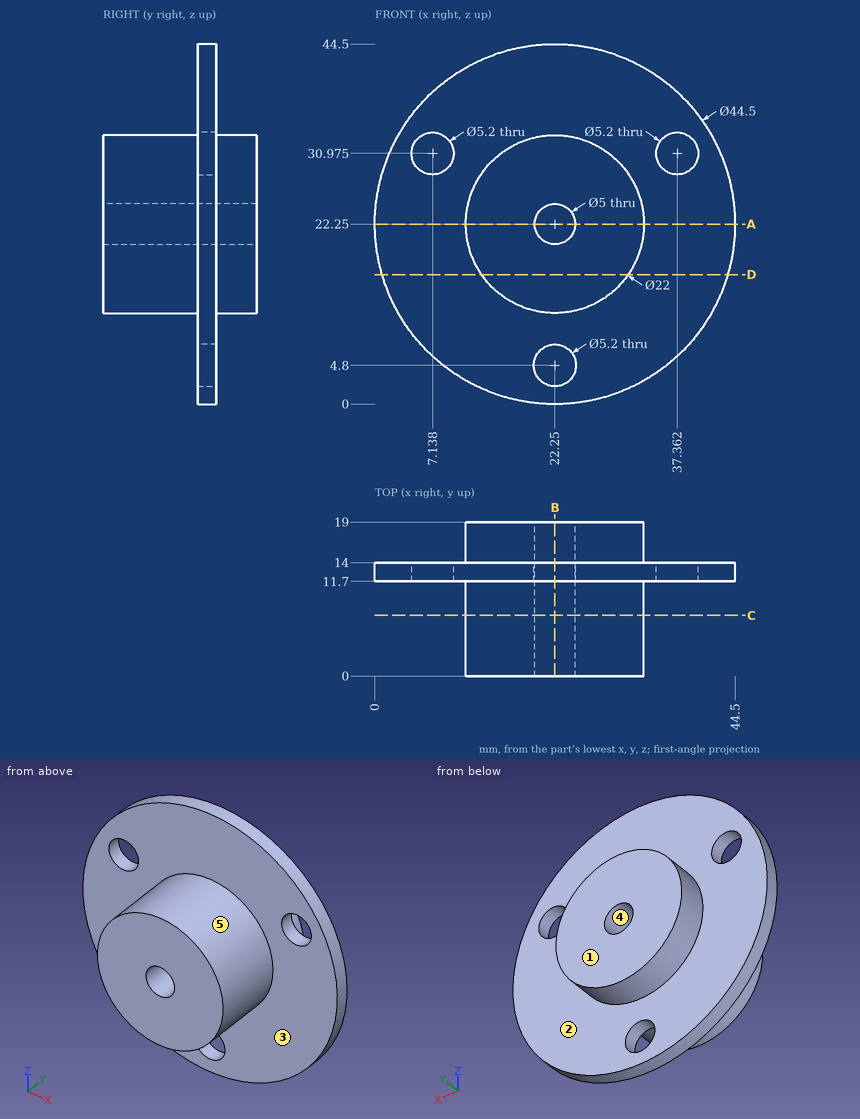
Job drawing, mm, ordinate dimensions from the low corner. One solid piece. A direction names the side the tool comes from. Give positions to 0.01 mm unless a question says otherwise; leave off trailing zeros. Order: outer loops, then holes, each group sorted by start corner. A loop starts at its lowest first (then second) coordinate and runs counter-clockwise, first axis right, second up. Notation, with made-up numbers: (52, 2) - (94, 2) arc R26 ccw to (94, 32) - close; hole circle Ø5 at (26.25, -40). An arc over 180 degrees is marked (long way). Return JSON: item names as keys, results as strings.
1) Flat gauge pins, fed straight in: P1, Ø6, axis at y = 6, z = 22, coming from the +X side; P2, Ø2, axis at y = 15.5, z = 31.5, coming from the -X side; P3, Ø10, axis at x = 10.5, y = 12.5, coming from the +Z side; P4, Ø8, axis at x = 22.25, z = 22.25, coming from the -Y side. Where does each tip first touch, or does it go through?
Geometry says:
{"P1": "x = 33.25", "P2": "x = 14.97", "P3": "z = 43.45", "P4": "y = 0"}
2) Cut at A-A, the plane z = 22.25. Give the cut face in (x, y).
Geometry says:
{"outline": "(0, 11.7) - (11.25, 11.7) - (11.25, 0) - (19.75, 0) - (19.75, 19) - (11.25, 19) - (11.25, 14) - (0, 14) - close; (24.75, 0) - (33.25, 0) - (33.25, 11.7) - (44.5, 11.7) - (44.5, 14) - (33.25, 14) - (33.25, 19) - (24.75, 19) - close"}
3) Pull direction Z, two halves, no side cores. Call the marked faces 3, 4 and 5: pulls with the +Z half, pulls with the -Z half, needs draft (parallel to the pull), parting line crosses it, or undercut.
Geometry says:
{"face 3": "needs draft", "face 4": "undercut", "face 5": "parting line crosses it"}
4) 3-axis set-ups, long thin cutter, end or side, ignore diameter. For the marked faces 1 and 2: which of +Z, -Z, +X, -X, +Y, -Y reach the whole face in a straight line?
Geometry says:
{"face 1": "+Z, -Z, +X, -X, +Y", "face 2": "+Y"}
5) Cut at D-D, the plane z = 16. Give the cut face in (x, y).
Geometry says:
{"outline": "(0.9, 11.7) - (13.2, 11.7) - (13.2, 0) - (31.3, 0) - (31.3, 11.7) - (43.6, 11.7) - (43.6, 14) - (31.3, 14) - (31.3, 19) - (13.2, 19) - (13.2, 14) - (0.9, 14) - close"}
6) Cut at B-B, the plane x = 22.25. Give the cut face in (y, z).
Geometry says:
{"outline": "(0, 11.25) - (11.7, 11.25) - (11.7, 7.4) - (14, 7.4) - (14, 11.25) - (19, 11.25) - (19, 19.75) - (0, 19.75) - close; (0, 24.75) - (19, 24.75) - (19, 33.25) - (14, 33.25) - (14, 44.5) - (11.7, 44.5) - (11.7, 33.25) - (0, 33.25) - close; (11.7, 0) - (14, 0) - (14, 2.2) - (11.7, 2.2) - close"}
7) Cut at C-C, the plane y = 7.5. Give the cut face in (x, z), plus the area to 4 significant figures.
Geometry says:
{"outline": "circle Ø22 at (22.25, 22.25); hole circle Ø5 at (22.25, 22.25)", "area": "360.5 mm²"}
8) Probe line 1 (Z direction, x = 22.5, y = 13.25); line 2 (Y direction, x = 33, z = 35); line 3 (X direction, y = 5, z = 20). List the from-to ranges inside material, lowest first. Write a range as from..to.
Geometry says:
{"line 1": "0..2.21, 7.39..19.76, 24.74..44.5", "line 2": "11.7..14", "line 3": "11.48..21.16, 23.34..33.02"}
